Geometry: final body of the model. Coordinates: model frame, mm. A direction names the side the tool comes from. Give positions to 0.01 mm unless a question says otherwise; leave off trailing zeros. Order: outer loops, then holes, each group sorted by start corner. A loop starts at its lowest first (then second) coordinate and runs counter-clockwise, first axis right, second up. Notation, with made-up numbers: (-28.75, 79) -> (13.25, 79) arc R37 ccw to (13.25, 116) -> close; hole circle Ø5 at (63.25, 38.5). An arc over 180 degrees is marked (long way). One line per question, with ' | ' between items.
from build123d import *

# Parameters (mm, degrees)
F0_W     = 1.5
F0_H     = 3
F1_DEPTH = 0.3
F2_DEPTH = 0.6
F3_R     = 4.75
F4_DEPTH = 2.3
F5_SIZE  = 2.29999
F6_SIZE  = 0.29999


# Not quite as in the source:
# - a fillet or chamfer is up to 0.001 mm smaller than in the source, because OpenCascade refuses the exact size


with BuildPart() as f1:
    # F0 (on Front) → F1 (new body)
    with BuildSketch(Plane.XZ):
        with BuildLine():
            Line((8.75, -6), (8.75, 6))
            Line((8.75, 6), (6.3639610307, 6))
            ThreePointArc((6.3639610307, 6), (0, 10.5), (-6.3639610307, 6))
            Line((-6.3639610307, 6), (-8.75, 6))
            Line((-8.75, 6), (-8.75, -6))
            Line((-8.75, -6), (-5, -6))
            Line((-5, -6), (-5, -3))
            Line((-5, -3), (5, -3))
            Line((5, -3), (5, -6))
            Line((5, -6), (8.75, -6))
        make_face()
        with Locations((-6.75, 0)):
            Rectangle(F0_W, F0_H, mode=Mode.SUBTRACT)
        with Locations((6.75, 0)):
            Rectangle(F0_W, F0_H, mode=Mode.SUBTRACT)
        with Locations((-6.75, 0)):
            Rectangle(F0_W, F0_H)
        with Locations((6.75, 0)):
            Rectangle(F0_W, F0_H)
    extrude(amount=F1_DEPTH)

    # F0 (on Front) → F2 (join)
    with BuildSketch(Plane.XZ):
        with Locations((-6.75, 0)):
            Rectangle(F0_W, F0_H)
        with Locations((6.75, 0)):
            Rectangle(F0_W, F0_H)
    extrude(amount=F2_DEPTH)

    # F3 (on face) → F4 (join)
    with BuildSketch(Plane.XZ.offset(0.3)):
        with Locations((0, 3.75)):
            Circle(F3_R)
    extrude(amount=F4_DEPTH)

    # F5 (size 2.3 in the source; OpenCascade refuses exactly that, so slightly less here)
    f5_edges = [f1.edges().sort_by_distance(p)[0] for p in [
        (-4.75, -2.6, 3.75),
    ]]
    chamfer(f5_edges, length=F5_SIZE)

    # F6 (size 0.3 in the source; OpenCascade refuses exactly that, so slightly less here)
    f6_edges = [f1.edges().sort_by_distance(p)[0] for p in [
        (-6.75, -0.6, -1.5),
        (-6.75, -0.6, 1.5),
        (6.75, -0.6, -1.5),
        (6.75, -0.6, 1.5),
        (-5, -0.15, -6),
        (-8.75, -0.15, -6),
        (5, -0.15, -6),
        (8.75, -0.15, -6),
        (8.75, -0.15, 6),
        (-8.75, -0.15, 6),
    ]]
    chamfer(f6_edges, length=F6_SIZE)


solid = f1.part
1) Pull-direction query (X, two-part tool) for faces 4 (the flat face through (-0.1, -0.3, -1.3)), 5 (the cylindrical face through (0.12, -0.15, 10.5)), 6 (the flat face through (0, 0, 2)); classes: +X half, -X half, draft (parallel to the pull), parting line (faces both ways), or undercut.
Check result:
face 4: undercut | face 5: parting line | face 6: draft
2) Material intervals for probe 1 along X at (y, z) = (-0.35, 0.5); probe 2 along Y at (x, z) = (7, -2.5); probe 3 along X at (y, z) = (-1.3, 6.25), sorted ascending. Write a range as from..to.
Check result:
probe 1: x = -7.5..-6, -3.4..3.4, 6..7.5 | probe 2: y = -0.3..0 | probe 3: x = -2.8..2.8
3) Section C-C on y = -1. Return loops of the section in (x, z), plus the area to 3 significant figures.
Check result:
outline: circle Ø8.1 at (0, 3.75) | area: 51.5 mm^2
4) Set-up query: faces 1 (the flat face through (-7, -0.6, 0)), 2 (the flat face through (7, -0.6, 0)), 3 (the flat face through (0, -2.6, 4)). Return all of +Z, -Z, +X, -X, +Y, -Y with unobstructed straight access to the full face (end or side cutting, diameter ignored); none if empty.
Check result:
face 1: +Z, -Z, -X, -Y | face 2: +Z, -Z, +X, -Y | face 3: +Z, -Z, +X, -X, -Y
5) Contact query for flat-ended pins moving along their axis: pin 1 Ø5 at (x, z) = (6, 1) entering from -Y; pin 2 Ø1.6 at (x, z) = (-6.5, 0) entering from -Y. Output: stop coordinate, or through.
Check result:
pin 1: stops at y = -0.95 | pin 2: stops at y = -0.6
6) Section D-D on y = -2.2. Return loops of the section in (x, z).
Check result:
outline: circle Ø5.7 at (0, 3.75)
